Could you check a few things on this drawing? It's one solid part, dimensions in mm from its lowest x, y, z. A direction names the side the tool comes from. Give positions to 0.01 mm unless a question says otherwise; leave off trailing zeros. Loops run counter-clockwise (first coordinate to the right, second up) from the corner with the lowest first, then second, coordinate; pieces in that order, holes last. Notation, with made-up numbers: M 78.5,26 L 83.5,26 A19 cw 83.5,56 Z; hole C 9,68.25 d4. An arc over 180 degrees is marked long. Answer in a Markdown table with one row per item. Add a question column.
1. Which directions (+Z, -Z, +X, -X, +Y, -Y) give clear straight access to the entire face, cutting with the end or side of a thin tool? Please do the marked faces 1 and 2.
2. I'm going to push flat-ended pins straight in: pin 1 Ø2 at (y, z) = (2.5, 3) entering from -X; pin 2 Ø4 at (x, y) = (3.5, 6.5) entering from -Z; pin 3 Ø3 at (x, y) = (2.5, 8) entering from +Z. Where does each tip first touch, or does it pass through?
3. If we section it at A-A on z = 3.5: List the corners of the cut face in (x, y) for me, then the cut area to 3 significant figures.
4. If we section it at B-B on x = 3.5: List the corners of the cut face in (y, z) for me.
5. I need wall thicknesses on line 1 along Y through (x, z) = (6.5, 2.5); line 2 along X through (y, z) = (4.5, 3.5); line 3 along Z through (x, y) = (1.75, 8.75). Which ranges of each line are inside material? Lowest first, please. Write a range as from..to.
6. If we section it at C-C on y = 8: List the corners of the cut face in (x, z) for me, then the cut area to 3 significant figures.
7. If we section it at D-D on x = 1: List the corners of the cut face in (y, z) for me.
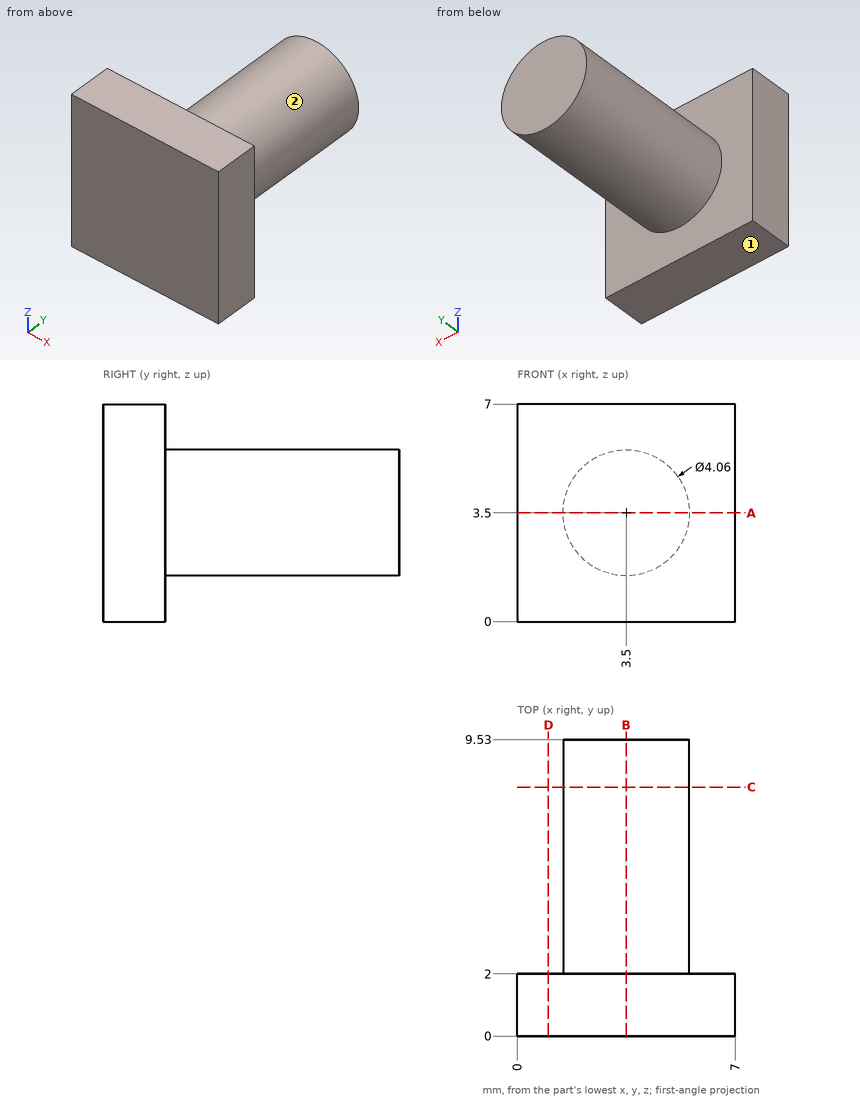
Results:
| question | item | result |
|---|---|---|
| 1 | face 1 | -Z, +X, -X, +Y, -Y |
| 1 | face 2 | +Y |
| 2 | pin 1 | x = 0 |
| 2 | pin 2 | z = 1.47 |
| 2 | pin 3 | z = 5.53 |
| 3 | outline | M 0,0 L 7,0 L 7,2 L 5.53,2 L 5.53,9.53 L 1.47,9.53 L 1.47,2 L 0,2 Z |
| 3 | area | 44.6 mm2 |
| 4 | outline | M 0,0 L 2,0 L 2,1.47 L 9.53,1.47 L 9.53,5.53 L 2,5.53 L 2,7 L 0,7 Z |
| 5 | line 1 | 0..2 |
| 5 | line 2 | 1.47..5.53 |
| 5 | line 3 | 2.47..4.53 |
| 6 | outline | C 3.5,3.5 d4.06 |
| 6 | area | 12.9 mm2 |
| 7 | outline | M 0,0 L 2,0 L 2,7 L 0,7 Z |
